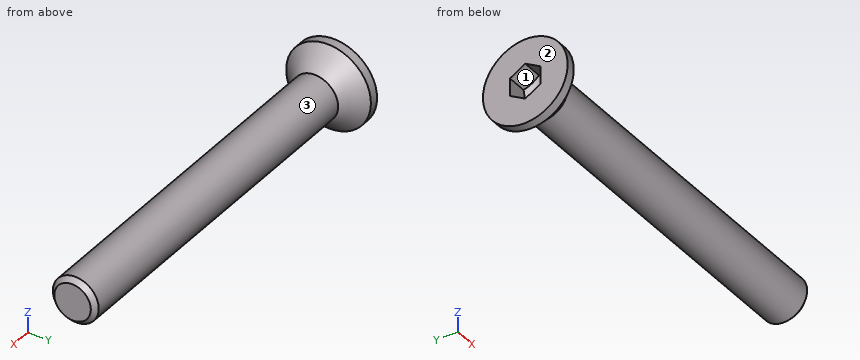
Autodesk Inventor part; units mm, degrees
ref_plane "Work Plane1" through (104.775, 0, 0) normal (0, 0, -1) x (1, 0, 0)
ref_plane "YZ Plane" through (0, 0, 0) normal (1, 0, 0) x (0, 1, 0)
ref_plane "XZ Plane" through (0, 0, 0) normal (0, 1, 0) x (-1, 0, 0)
sketch "Esquisse1" plane through (0, 0, 0) normal (0, 0, 1) x (1, 0, 0)
  line L0 (25, 0) -> (25, 1.5)
  line L1 (25, 1.5) -> (7, 1.5)
  line L2 (7, 1.5) -> (6.6933, 1.5)
  line L3 (0, 2.77) -> (0, 1.1547)
  line L4 (0, 1.1547) -> (1.3, 1.1547)
  line L5 (1.3, 1.1547) -> (1.9667, 0)
  line L6 (1.9667, 0) -> (25, 0)
  line L7 (0, 2.77) -> (0.59, 2.77)
  line L8 (0.59, 2.77) -> (1.86, 1.5)
  line L9 (6.6933, 1.5) -> (1.86, 1.5)
  line L10 (7, 1.5) -> (1.86, 1.5) construction
  line L11 (1.86, 1.5) -> (1.86, 1.5)
  line L12 (-5, 0) -> (30, 0)
  line L13 (0, -0.554) -> (0, 3.324)
  dimension "d0" = 25
  dimension "d1" = 18
  dimension "d2" = 1.3
  dimension "d3" = 3
  dimension "d6" = 1.86
  dimension "d7" = 45
  dimension "d8" = 2.3094
  dimension "d9" = 60
  dimension "d10" = 5.54
  dimension "d11" = 3
  dimension "d12" = 0.3067
revolve "Corps" add sketch "Esquisse1" angle 360 about axis through (1.9667, 0, 0) along (1, 0, 0) contours L6 L5 L4 L3 L7 L8 L9 L2 L1 L0
sketch "Esquisse2" plane through (0, 0, 0) normal (-1, 0, 0) x (0, 0, 1)
  circle A0 centre (0, 0) radius 1.1547
  line L0 (0, -3.878) -> (0, 3.878)
  line L1 (-3.878, 0) -> (3.878, 0)
  line L2 (1.1547, 0) -> (0.5774, -1)
  line L3 (0.5774, -1) -> (-0.5774, -1)
  line L4 (-0.5774, -1) -> (-1.1547, 0)
  line L5 (-1.1547, 0) -> (-0.5774, 1)
  line L6 (-0.5774, 1) -> (0.5774, 1)
  line L7 (0.5774, 1) -> (1.1547, 0)
  point P0 (0, 1.1547)
extrude "Rainure" add sketch "Esquisse2" against normal up to next contours L7 A0 | A0 L2 | L6 L0 A0 | A0 L0 L3 | L0 L6 A0 | A0 L3 L0 | L4 A0 | A0 L5
thread "Filetage"
chamfer "Chanfrein1" distance 0.3067 distance2 0.3067 1 edges at (25, -1.5, 0) measured on face at (25, 0.0871, 0.3876)
ref_plane "Work Plane1" through (104.775, 0, 0) normal (0, 0, -1) x (1, 0, 0)
equation "\"d15\" = GEL"
equation "\"d17\" = -0.5 * SPD + 0.5 * GD"
equation "\"d18\" = GUL"
equation "\"d0\" = NLG"
equation "\"d1\" = GEL"
equation "\"d2\" = INTI"
equation "\"d3\" = GD"
equation "\"d6\" = KOH"
equation "\"d7\" = 0.5 * SEWI"
equation "\"d8\" = 1.1547 * SW"
equation "\"d10\" = KOD"
equation "\"d11\" = BDM"
equation "\"d12\" = GAL"
equation "\"NLG\" = 25"
equation "\"INTI\" = 1.3"
equation "\"GEL\" = 18"
equation "\"GAL\" = 0.61345 * PTC"
equation "\"KOH\" = 1.86"
equation "\"KOD\" = 5.54"
equation "\"GUL\" = 0.61345 * PTC"
equation "\"SPD\" = NND - 1.2269 * PTC"
equation "\"BDM\" = NND"
equation "\"GD\" = NND"
equation "\"SEWI\" = 90deg"
equation "\"SW\" = 2"
equation "\"TOA\" = 30deg"
equation "\"GD1\" = THREADDIA - 1.2269 * PTC"
equation "\"EPV\" = 3.36"
equation "\"THREADDIA\" = 3"
equation "\"PTC\" = 0.5"
equation "\"NND\" = 3"
equation "\"E0\" = 2.31"
equation "\"THREADDESC\" = 1.2345"
properties part number "ISO 10642 - M3 x  25" material "Acier"
For this review, take the finished solid that the model builds, in its own axes (mm). Face numbers are marked on the shaded views. Coordinates: 2 decimals unless noted, no trailing zeros. Loops run counter-clockwise (first coordinate to the right, second up) from the corner with the lowest first, then second, coordinate; pieces in that order, holes last.
1. For line 1 (Y direction, x = 12.75, z = 0.8); line 2 (Y direction, x = 3.25, z = 1.15); line 3 (X direction, y = -1.75, z = -1.4), list the stretches that pass through material, from the lowest coordinate up.
2. Add section A-A, the plane x = 8.5. Give the boundary of the cut face in (y, z), then the cut area to 3 significant figures.
3. Insertion check: P1, Ø2, axis at x = 18, y = -1, coming from the +Z side; P2, Ø1, axis at x = 14.5, z = 0, coming from the -Y side. Each pin has a flat end and moves straight along its axis. Give the tip position at first contact, or say it passes through.
4. Mouldability with a two-part tool opening along Y and no side actions: class the marked faces 1, 2 and 3 as +Y half, -Y half, draft (parallel to the pull), parting line (faces both ways), or undercut.
Result:
1. line 1: y = -1.27 to 1.27
1. line 2: y = -0.96 to 0.96
1. line 3: x = 0 to 1.12
2. outline: circle Ø3 at (0, 0)
2. area: 7.07 mm2
3. P1: stops at z = 1.5
3. P2: stops at y = -1.5
4. face 1: undercut
4. face 2: draft
4. face 3: parting line
